Geometry check sheet. Reference: the model listing, model coordinates, mm. Round coordinates to 2 decimals unless told otherwise and drop trailing zeros. Loops run counter-clockwise (first coordinate to the right, second up) from the corner with the lowest first, then second, coordinate; pieces in that order, holes last. Notation, with made-up numbers: (73.25, 50.25) - (102.25, 50.25) arc R27 cw to (102.25, 80.25) - close; hole circle Ø9 at (17.25, 38.5). An arc over 180 degrees is marked (long way). Answer as CSV lines item,"result". Start each with the question number.
1) Cross-section at C-C on x = 45.5. Record the boundary of the cut face in (y, z), and give its area (3 significant figures).
2) Cross-section at B-B on z = 2.95. Record the boundary of the cut face in (x, y).
3) Cross-section at A-A on y = 33. Record the boundary of the cut face in (x, z).
4) Depth check by flat-ended pin: P1, Ø2, axis at x = 49, z = 3, coming from the -Y side. Enter the tip coordinate at first touch or a pass-through.
5) Thickness scan on line 1 along X through (y, z) = (50, 2.1); line 2 along Y through (x, z) = (26, 0.9). Record the ranges inside material, lowest first.
from build123d import *

# Parameters (mm, degrees)
F1_DEPTH = 3.75
F2_W     = 3.75
F2_H     = 50
F3_DEPTH = 3.75


with BuildPart() as f1:
    # F0 (on Top) → F1 (new body)
    with BuildSketch(Plane.XY):
        Polygon((20, -23.677632), (20, -16.177632), (52.782, -16.177632), (52.782, -23.677632), (72.782, -23.677632), (72.782, -16.177632), (72.782, 183.822368), (0, 183.822368), (0, -16.177632), (0, -23.677632), align=None)
    extrude(amount=F1_DEPTH)

    # F2 (on face) → F3 (cut)
    with BuildSketch(Plane.XY.offset(3.75)):
        with Locations((36.391, 50.822368)):
            Rectangle(F2_W, F2_H)
        with Locations((36.391, 133.822368)):
            Rectangle(F2_W, F2_H)
    extrude(amount=-F3_DEPTH, mode=Mode.SUBTRACT)


solid = f1.part
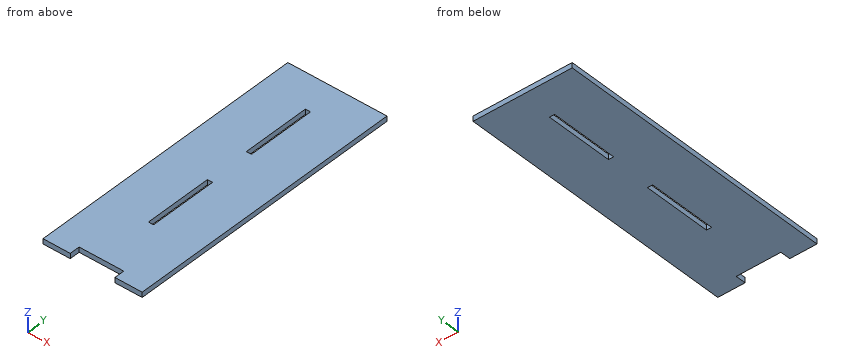
Answer block:
1,outline,"(-16.18, 0) - (183.82, 0) - (183.82, 3.75) - (-16.18, 3.75) - close"
1,area,"750 mm^2"
2,outline,"(0, -23.68) - (20, -23.68) - (20, -16.18) - (52.78, -16.18) - (52.78, -23.68) - (72.78, -23.68) - (72.78, 183.82) - (0, 183.82) - close; hole (34.52, 25.82) - (38.27, 25.82) - (38.27, 75.82) - (34.52, 75.82) - close; hole (34.52, 108.82) - (38.27, 108.82) - (38.27, 158.82) - (34.52, 158.82) - close"
3,outline,"(0, 0) - (34.52, 0) - (34.52, 3.75) - (0, 3.75) - close; (38.27, 0) - (72.78, 0) - (72.78, 3.75) - (38.27, 3.75) - close"
4,P1,"stops at y = -16.18"
5,line 1,"x = 0 to 34.52, 38.27 to 72.78"
5,line 2,"y = -16.18 to 183.82"
